Check sheet for the modelled part. Datum: model origin and axes. Units: mm. A direction names the side the tool comes from. Give positions to 0.01 mm unless a question says otherwise; leave off trailing zeros. Write each loop counter-clockwise with the first axis right and the second up, starting at its lowest first coordinate (ties: lowest second). Pieces come first, ordered by that corner, then holes. Notation, with made-up numbers: (75, 76.5) -> (108, 76.5) arc R13 cw to (108, 99.5) -> close; hole circle Ø5 at (-27.75, 80). An arc over 180 degrees is marked (long way). Answer as a JSON object with one key per item and string values.
from build123d import *

# Parameters (mm, degrees)
F0_R     = 5.5
F1_DEPTH = 9
F3_START = -17.3870930076
F2_W     = 59
F2_H     = 9
F3_DEPTH = 8.9999069924
F5_R     = 7
F6_DEPTH = 9


with BuildPart() as f1:
    # F0 (on Top) → F1 (new body)
    with BuildSketch(Plane.XY):
        with BuildLine():
            Line((46, 17.3870930076), (-13, 17.3870930076))
            Line((-13, 17.3870930076), (-13, 2.3870930076))
            ThreePointArc((-13, 2.3870930076), (-9.1923881554, -6.8052951478), (0, -10.6129069924))
            Line((0, -10.6129069924), (33, -10.6129069924))
            ThreePointArc((33, -10.6129069924), (42.1923881554, -6.8052951478), (46, 2.3870930076))
            Line((46, 2.3870930076), (46, 17.3870930076))
        make_face()
        with Locations((0, 2.3870930076)):
            Circle(F0_R, mode=Mode.SUBTRACT)
        with Locations((33, 2.3870930076)):
            Circle(F0_R, mode=Mode.SUBTRACT)
    extrude(amount=F1_DEPTH)

    # F2 (on Front) → F3 (join)
    with BuildSketch(Plane.XZ.offset(F3_START)):
        with Locations((16.5, 4.5)):
            Rectangle(F2_W, F2_H)
        Polygon((46, 9), (46, 0), (62.2267983854, 53.5452626646), (41.3173237145, 74.4547373354), (-13, 9), align=None)
    extrude(amount=-F3_DEPTH)

    # F5 (on offset) → F6 (join)
    with BuildSketch(Plane(origin=(57.886030525, 0, 57.886030525), x_dir=(0, 1, 0), z_dir=(0.7071067812, 0, 0.7071067812))):
        with BuildLine():
            Line((-2.613, -6.1387727793), (26.387, -6.1387727793))
            Line((26.387, -6.1387727793), (26.387, 23.4316898824))
            Line((26.387, 23.4316898824), (-2.613, 23.4316898824))
            ThreePointArc((-2.613, 23.4316898824), (-12.4976966965, 8.6464585515), (-2.613, -6.1387727793))
        make_face()
        with Locations((3.5023033035, 8.6464585515)):
            Circle(F5_R, mode=Mode.SUBTRACT)
    extrude(amount=-F6_DEPTH)


solid = f1.part
1. Sectioned sample at B-B, the plane x = 19.5. Enter the section's corners in (y, z).
Determined:
{"outline": "(-10.61, 0) -> (26.39, 0) -> (26.39, 48.16) -> (17.39, 48.16) -> (17.39, 9) -> (-10.61, 9) -> close"}
2. Mould release check, pull along Z, two halves, no side actions. Record for faces 4 (the face through (27.505, 2.629, 4.437)), 5 (the face through (16, 4, 9)), 6 (the face through (54, 21.8, 26.4)): released by +Z, released by -Z, zero draft, split by the parting line, or undercut.
Determined:
{"face 4": "zero draft", "face 5": "undercut", "face 6": "released by -Z"}
3. Sectioned sample at A-A, the plane y = -4.5. Enter the section's corners in (x, z).
Determined:
{"outline": "(-11.03, 0) -> (44.03, 0) -> (44.03, 9) -> (-11.03, 9) -> close; (35.61, 67.43) -> (55.21, 47.84) -> (61.57, 54.2) -> (41.98, 73.8) -> close"}
4. Go/stop test with flat-tipped pins: P1, Ø4.5, axis at y = 8, z = 3.5, coming from the +X side; P2, Ø9, axis at x = 33, y = 2.39, coming from the -Z side; P3, Ø2.5, axis at x = 12, z = 4.5, coming from the -Y side. Record where each tip stops, or that it passes through.
Determined:
{"P1": "x = 46", "P2": "z = 65.54", "P3": "y = -10.61"}
5. Access from +Z, -Z, +X, -X, +Y, -Y to the whole of each face (thin tool, end or side, straight path). Record for faces 1 (the face through (45.262, 10.993, 57.782)), 2 (the face through (16, -10.613, 4)), 3 (the face through (42.091, -6.906, 4.437)).
Determined:
{"face 1": "-X, -Y", "face 2": "+Z, -Z, +X, -X, -Y", "face 3": "-Z, +X, -Y"}
6. Sectioned sample at C-C, the plane z = 23. Enter the section's corners in (x, y), plus the area to 3 significant figures.
Determined:
{"outline": "(-1.38, 17.39) -> (52.97, 17.39) -> (52.97, 26.39) -> (-1.38, 26.39) -> close", "area": "489 mm^2"}
7. Scan lines: L1, parallel to Y at x = 33, z = 3.5; L2, parallel to Z at x = -0.5, y = 11; L3, parallel to Y at x = 38.5, z = 56. Record each from-to range of solid material in increasing order. Write a range as [from, to].
Determined:
{"L1": "[-10.61, -3.11], [7.89, 26.39]", "L2": "[0, 9]", "L3": "[17.39, 26.39]"}
